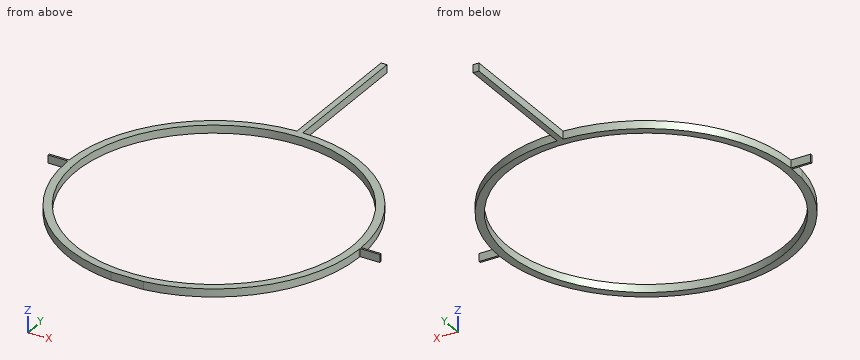
from build123d import *

# Parameters (mm, degrees)
F0_R     = 35
F1_DEPTH = 1


with BuildPart() as f1:
    # F0 (on Top) → F1 (new body, symmetric)
    with BuildSketch(Plane.XY):
        with BuildLine():
            Line((-1.5, 72), (-1.5, 36.969582))
            ThreePointArc((-1.5, 36.969582), (-26.514279, 25.806841), (-36.996623, 0.499897))
            Line((-36.996623, 0.499897), (-41.996623, 0.499897))
            Line((-41.996623, 0.499897), (-41.986487, 0))
            Line((-41.986487, 0), (-36.968242, 0))
            Line((-36.968242, 0), (-36.702311, -4.684058))
            ThreePointArc((-36.702311, -4.684058), (-25.811947, -26.509307), (-3.704199, -36.814113))
            Line((-3.704199, -36.814113), (4.491361, -36.726389))
            ThreePointArc((4.491361, -36.726389), (27.539081, -24.710302), (36.996621, -0.5))
            Line((36.996621, -0.5), (36.996621, 0))
            Line((36.996621, 0), (41.996621, 0))
            Line((41.996621, 0), (41.996621, 0.5))
            Line((41.996621, 0.5), (36.996621, 0.5))
            ThreePointArc((36.996621, 0.5), (25.985573, 26.339134), (0, 37))
            Line((0, 37), (0, 72))
            Line((0, 72), (-1.5, 72))
        make_face()
        Circle(F0_R, mode=Mode.SUBTRACT)
    extrude(amount=F1_DEPTH, both=True)


solid = f1.part
The model under review builds one solid part; all positions refer to its coordinate system, in mm. Round coordinates to 2 decimals unless told otherwise and drop trailing zeros. Loops run counter-clockwise (first coordinate to the right, second up) from the corner with the lowest first, then second, coordinate; pieces in that order, holes last. Notation, with made-up numbers: (58.25, 62) -> (110.25, 62) arc R14 cw to (110.25, 82) -> close; hole circle Ø4 at (2.5, 88). An arc over 180 degrees is marked (long way). Return JSON: item names as keys, results as strings.
(1) Add section A-A on x = 8.5. Write out the cut boundary in (y, z), plus the area to 3 significant figures.
Solved:
{"outline": "(-36.01, -1) -> (-33.95, -1) -> (-33.95, 1) -> (-36.01, 1) -> close; (33.95, -1) -> (36.01, -1) -> (36.01, 1) -> (33.95, 1) -> close", "area": "8.23 mm2"}
(2) Add section B-B on y = -2. Write out the cut boundary in (x, z).
Solved:
{"outline": "(-36.85, -1) -> (-34.94, -1) -> (-34.94, 1) -> (-36.85, 1) -> close; (34.94, -1) -> (36.95, -1) -> (36.95, 1) -> (34.94, 1) -> close"}
(3) For pin 1 (4 mm diameter, centred on x = 30.5, y = -7.5, fed in from +Z); pin 2 (0.6 mm diameter, centred on x = -40.5, z = 0.5, fed in from -Y); pin 3 (0.6 mm diameter, centred on y = 50.5, z = 0, fed in from -X), all flat-tipped, find the tip position at first contact; note any pin that passes through.
Solved:
{"pin 1": "through", "pin 2": "y = 0", "pin 3": "x = -1.5"}
(4) Add section D-D on y = 47. Write out the cut boundary in (x, z), plus the area to 3 significant figures.
Solved:
{"outline": "(-1.5, -1) -> (0, -1) -> (0, 1) -> (-1.5, 1) -> close", "area": "3.00 mm2"}
(5) For line 1 (X direction, y = 10, z = 0.2); line 2 (X direction, y = 45, z = 0.1); line 3 (Y direction, x = -29, z = -0.4), list the stretches that pass through material, from the lowest coordinate up.
Solved:
{"line 1": "-35.62 to -33.54, 33.54 to 35.62", "line 2": "-1.5 to 0", "line 3": "-22.98 to -19.6, 19.6 to 22.98"}
(6) Add section C-C on z = -0.35. Write out the cut boundary in (x, y), plus the area to 3 significant figures.
Solved:
{"outline": "(-42, 0.5) -> (-41.99, 0) -> (-36.97, 0) -> (-36.7, -4.68) arc R37 ccw to (-3.7, -36.81) -> (4.49, -36.73) arc R37 ccw to (37, -0.5) -> (37, 0) -> (42, 0) -> (42, 0.5) -> (37, 0.5) arc R37 ccw to (0, 37) -> (0, 72) -> (-1.5, 72) -> (-1.5, 36.97) arc R37 ccw to (-37, 0.5) -> close; hole circle Ø70 at (0, 0)", "area": "508 mm2"}
